```python
from build123d import *

# Parameters (mm, degrees)
CYLINDER_W     = 130
CYLINDER_H     = 300
CYLINDER_ANGLE = 180
SPHERE_ANGLE   = 180
CONE_ANGLE     = 180
FILLET_R       = 55


with BuildPart() as cylinder:
    # Cylinder → Cylinder (revolve)
    with BuildSketch(Plane(origin=(0, 500, 0), x_dir=(1, 0, 0), z_dir=(0, 0, -1))):
        with Locations((65, 150)):
            Rectangle(CYLINDER_W, CYLINDER_H)
    revolve(axis=Axis((0, 500, 0), (0, -1, 0)), revolution_arc=CYLINDER_ANGLE)


with BuildPart() as sphere:
    # Sphere → Sphere (revolve)
    with BuildSketch(Plane(origin=(0, 500, 0), x_dir=(1, 0, 0), z_dir=(0, 0, -1))):
        with BuildLine():
            ThreePointArc((0, -130), (91.923882, -91.923882), (130, 0))
            Line((130, 0), (0, 0))
            Line((0, 0), (0, -130))
        make_face()
    revolve(axis=Axis((0, 500, 0), (0, -1, 0)), revolution_arc=SPHERE_ANGLE)


with BuildPart() as fillet_body:
    # Cone → Cone (revolve)
    with BuildSketch(Plane(origin=(0, 0, 0), x_dir=(-1, 0, 0), z_dir=(0, 0, -1))):
        Polygon((0, 0), (15, 0), (130, 200), (0, 200), align=None)
    revolve(axis=Axis((0, 0, 0), (0, 1, 0)), revolution_arc=CONE_ANGLE)

    # Fusion: union Cylinder, Sphere
    add(cylinder.part)
    add(sphere.part)

    # Fillet
    fillet_edges = [fillet_body.edges().sort_by_distance(p)[0] for p in [
        (130, 350, 0),
    ]]
    fillet(fillet_edges, radius=FILLET_R)


solid = fillet_body.part
```
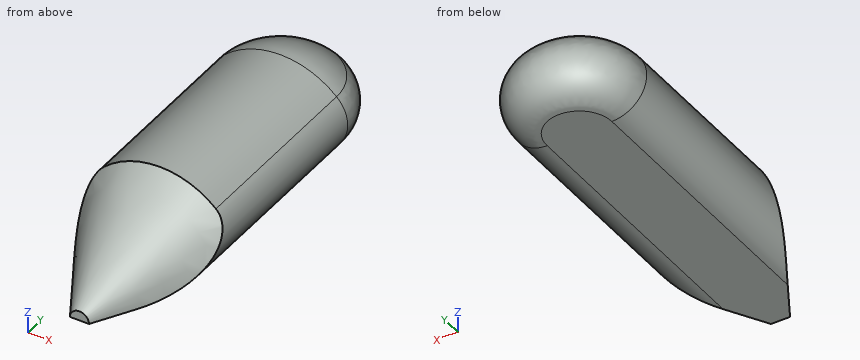
Geometry check sheet. Reference: the model listing, model coordinates, mm. Coordinates: 2 decimals unless noted, no trailing zeros. Loops run counter-clockwise (first coordinate to the right, second up) from the corner with the lowest first, then second, coordinate; pieces in that order, holes last. Notation, with made-up numbers: (19.25, 64) - (68.25, 64) arc R13 ccw to (68.25, 79) - close; hole circle Ø1 at (66.5, 35.5). An arc over 180 degrees is marked (long way). One line per item, written item: value. Start each with the question number.
(1) Depth check by flat-ended pin: P1, Ø4, axis at x = -82.5, z = 59, coming from the +Y side; P2, Ø2, axis at x = 74, z = 77.5, coming from the +Y side; P3, Ø12, axis at x = -38.5, z = 42, coming from the -Y side. Enter the tip coordinate at first touch or a pass-through.
(2) Cross-section at A-A on y = 488. Enter the section's corners in (x, z), plus the area to 3 significant figures.
(3) Material ranges on line 1 (X direction, y = 209.5, z = 34); line 2 (X direction, y = 277, z = 106.5); line 3 (Z direction, x = 46, y = 104), recorded low to high. Write a range as [from, to].
(4) Cross-section at B-B on y = 150. Enter the section's corners in (x, z), plus the area to 3 significant figures.
Results below:
1. P1: stops at y = 568.73
1. P2: stops at y = 570.24
1. P3: stops at y = 62.57
2. outline: (-88.38, 95.33) arc R55 ccw to (-50.99, 0) - (50.99, 0) arc R55 ccw to (88.38, 95.33) arc R130 ccw to start
2. area: 22,700 mm2
3. line 1: x = [-101.82, 101.82]
3. line 2: x = [-74.55, 74.55]
3. line 3: z = [0, 58.98]
4. outline: (-97.82, 26.15) arc R55 ccw to (-50.99, 0) - (50.99, 0) arc R55 ccw to (97.82, 26.15) arc R101.25 ccw to start
4. area: 15,300 mm2
